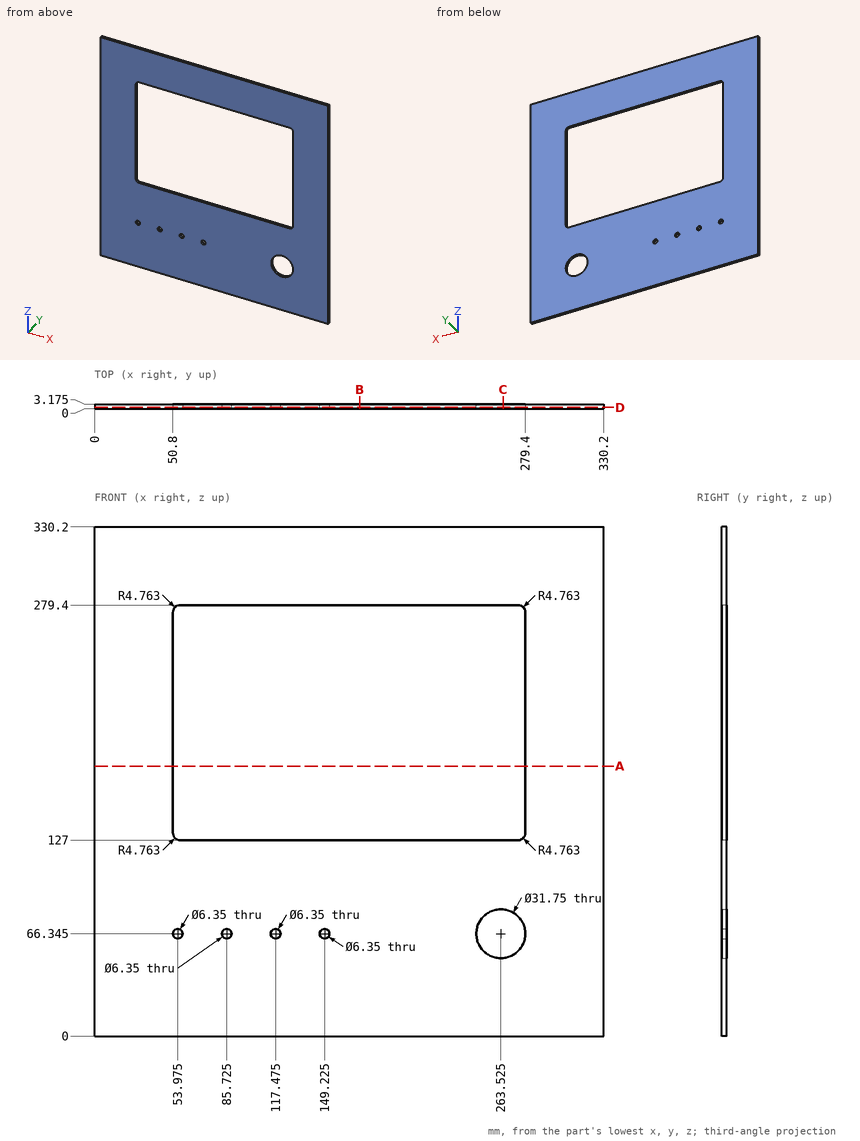
Print and shaded views of the part. All mm, measured from the part's lowest x, y and z. Coordinates: 2 decimals unless noted, no trailing zeros. Loops run counter-clockwise (first coordinate to the right, second up) from the corner with the lowest first, then second, coordinate; pieces in that order, holes last. Notation, with made-up numbers: (29.25, -22.5) - (81.25, -22.5) arc R22 ccw to (81.25, -13.5) - close; hole circle Ø5 at (-30.75, -39). An arc over 180 degrees is marked (long way). Use one line per item in the form item = value. Start each with the question number.
1) Drill centre lines: L1, parallel to X at y = 0.1, z = 264; L2, parallel to Z at x = 139, y = 0.35. Where is each one in solid material? Low to high. Write a range as from..to.
2) Band-saw the part on A-A (z = 175). Give the cut face in (x, y) (1 decimal).
3) Band-saw the part on C-C (x = 265). Give the cut face in (y, z) (1 decimal).
4) Flat gauge pin, fed straight in: pin 1 (5.5 mm diameter, centred on x = 149.22, z = 66.35, fed in from -Y). Where does the tip first touch, or does it go through?
5) Band-saw the part on D-D (y = 1). State how many separate pieces and enclosed holes the cut face has, and give its area (3 significant figures).
6) Band-saw the part on B-B (x = 172). Give the cut face in (y, z) (1 decimal).
Check values:
q1.L1 = 0..50.8, 279.4..330.2
q1.L2 = 0..127, 279.4..330.2
q2.outline = (0, 0) - (50.8, 0) - (50.8, 3.2) - (0, 3.2) - close; (279.4, 0) - (330.2, 0) - (330.2, 3.2) - (279.4, 3.2) - close
q3.outline = (0, 0) - (3.2, 0) - (3.2, 50.5) - (0, 50.5) - close; (0, 82.2) - (3.2, 82.2) - (3.2, 127) - (0, 127) - close; (0, 279.4) - (3.2, 279.4) - (3.2, 330.2) - (0, 330.2) - close
q4.pin_1 = through
q5.separate_pieces = 1
q5.enclosed_holes = 6
q5.area = 73,300 mm2
q6.outline = (0, 0) - (3.2, 0) - (3.2, 127) - (0, 127) - close; (0, 279.4) - (3.2, 279.4) - (3.2, 330.2) - (0, 330.2) - close
